Check sheet for the modelled part. Datum: model origin and axes. Units: mm. A direction names the side the tool comes from. Round coordinates to 2 decimals unless told otherwise and drop trailing zeros. Write each loop counter-clockwise with the first axis right and the second up, starting at its lowest first coordinate (ties: lowest second). Pieces come first, ordered by that corner, then holes. Notation, with made-up numbers: (86.5, 30) - (131.5, 30) arc R20 ccw to (131.5, 53) - close; hole circle Ø1 at (-26.5, -27.75). An arc over 180 degrees is marked (long way). Use one line per item in the form item = value. Start each with the question number.
1) Section check C-C (x = 10). Record the boundary of the cut face in (y, z) (1 decimal).
2) Draft check along Y on faces 4 (the face through (0, 477, 0)), 5 (the face through (0.03, 330.53, 24.14)), 6 (the face through (0, 0, 6)). Enter one of: +Y half, -Y half, draft (parallel to the pull), parting line (faces both ways), or undercut.
3) Set-up check for faces 1 (the face through (0.033, 439.75, 23.797)), 2 (the face through (11.26, 385.51, 34.1)), 3 (the face through (-11.46, 320.03, 4.19)): record each of +Z, -Z, +X, -X, +Y, -Y from which the full face is reachable in a straight line by a thin tool's end or side.
4) Scan lines: probe 1 along Z at (x, y) = (-3.5, 344); probe 2 along X at (y, z) = (83.5, 20); probe 3 along Z at (x, y) = (0, 378). Record each from-to range of solid material in increasing order.
5) Section check A-A (y = 385). Record the boundary of the cut face in (x, z).
6) Section check B-B (x = -8). Record the boundary of the cut face in (y, z) (1 decimal), then the cut area to 3 significant figures.
7) Gauge pin test, flat ends, axial feed: P1, Ø6, axis at x = 11.5, y = 437.5, coming from the +Z side; P2, Ø4, axis at x = -11.5, y = 246, coming from the +Z side; P3, Ø8, axis at x = -5.5, z = 46, coming from the +Y side; P4, Ø4, axis at x = 11, y = 244.5, coming from the -Z side. Record the tip position at first contact, or that the pin passes through.
from build123d import *

# Parameters (mm, degrees)
F1_DEPTH      = 15.08125
F1_DEPTH_BACK = 15.08125
F2_R          = 63.5
F3_R          = 22.225
F4_R          = 12.7


with BuildPart() as f1:
    # F0 (on Right) → F1 (new body, two sides)
    with BuildSketch(Plane.YZ) as f1_sk:
        Polygon((0, 14.2875), (0, 0), (323.85, 0), (323.85, 30.48), (446.0875, 30.48), (446.0875, 0), (508, 0), (508, 38.1), (482.6, 51.60542), (446.0875, 63.5), (323.85, 63.5), (25.4, 25.06916), align=None)
    extrude(amount=F1_DEPTH)
    extrude(f1_sk.sketch, amount=-F1_DEPTH_BACK)

    # F2
    f2_edges = [f1.edges().sort_by_distance(p)[0] for p in [
        (0, 25.4, 25.06916),
        (0, 323.85, 63.5),
        (0, 446.0875, 63.5),
        (0, 482.6, 51.60542),
    ]]
    fillet(f2_edges, radius=F2_R)

    # F3
    f3_edges = [f1.edges().sort_by_distance(p)[0] for p in [
        (0, 323.85, 30.48),
        (0, 446.0875, 30.48),
    ]]
    fillet(f3_edges, radius=F3_R)

    # F4
    f4_edges = [f1.edges().sort_by_distance(p)[0] for p in [
        (15.08125, 381.963359, 63.5),
        (-15.08125, 381.963359, 63.5),
        (15.08125, 384.96875, 30.48),
        (-15.08125, 384.96875, 30.48),
    ]]
    fillet(f4_edges, radius=F4_R)


solid = f1.part
Results are:
q1.outline = (0, 0) - (321.3, 0) - (321.3, 8.3) arc R24.8 cw to (346.1, 33) - (423.9, 33) arc R24.8 cw to (448.6, 8.3) - (448.6, 0) - (508, 0) - (508, 35.2) - (486.3, 46.8) arc R61 ccw to (476.6, 50.9) - (454.9, 58) arc R61 ccw to (436, 61) - (327.9, 61) arc R61 ccw to (320.1, 60.5) - (34.4, 23.7) arc R61 ccw to (18.4, 19.3) - (0, 11.5) - close
q2.face_4 = draft
q2.face_5 = undercut
q2.face_6 = -Y half
q3.face_1 = -Z, +X, -X
q3.face_2 = -Z, +X
q3.face_3 = -Z, -X
q4.probe_1 = 30.43 to 63.45
q4.probe_2 = -15.08 to 15.08
q4.probe_3 = 30.48 to 63.5
q5.outline = (-15.08, 43.18) arc R12.7 ccw to (-2.38, 30.48) - (2.38, 30.48) arc R12.7 ccw to (15.08, 43.18) - (15.08, 50.8) arc R12.7 ccw to (2.38, 63.5) - (-2.38, 63.5) arc R12.7 ccw to (-15.08, 50.8) - close
q6.outline = (0, 0) - (322.5, 0) - (322.5, 8.3) arc R23.5 cw to (346.1, 31.8) - (423.9, 31.8) arc R23.5 cw to (447.4, 8.3) - (447.4, 0) - (508, 0) - (508, 36.6) - (486.9, 47.9) arc R62.2 ccw to (476.9, 52.1) - (455.3, 59.1) arc R62.2 ccw to (436, 62.2) - (327.9, 62.2) arc R62.2 ccw to (320, 61.7) - (34.2, 24.9) arc R62.2 ccw to (17.9, 20.5) - (0, 12.9) - close
q6.area = 20,300 mm²
q7.P1 = 61.91
q7.P2 = 51.3
q7.P3 = 500.06
q7.P4 = 0
